from build123d import *

# Parameters (mm, degrees)
SKETCH1_R                    = 9
SKETCH1_R_2                  = 1
BOSS_EXTRUDE1_DEPTH          = 36
SKETCH5_W                    = 5
SKETCH5_H                    = 4.08502449
SKETCH5_W_2                  = 8
BOSS_EXTRUDE2_DEPTH          = 22
SKETCH7_W                    = 5
SKETCH7_H                    = 4.653899232
CUT_REVOLVE2_ANGLE           = 90
CUT_REVOLVE2_OTHER_WAY_ANGLE = 90
CIRPATTERN1_COUNT            = 15
SKETCH13_W                   = 5
SKETCH13_H                   = 16.616445935
SKETCH17_R                   = 2
CUT_EXTRUDE1_DEPTH           = 10
CUT_EXTRUDE2_DEPTH           = 23
CUT_EXTRUDE2_DEPTH_BACK      = 8
SKETCH20_R                   = 20.157813079
CUT_EXTRUDE3_DEPTH           = 36
FILLET1_R                    = 1


with BuildPart() as part:
    # Sketch1 → Boss-Extrude1 (new body)
    with BuildSketch(Plane.XY):
        Circle(SKETCH1_R)
        Circle(SKETCH1_R_2, mode=Mode.SUBTRACT)
    extrude(amount=BOSS_EXTRUDE1_DEPTH)

    # Sketch5 → Cut-Revolve1 (revolve, cut)
    with BuildSketch(Plane(origin=(0, 0, 0), x_dir=(0, 0, -1), z_dir=(1, 0, 0)), mode=Mode.PRIVATE) as cut_revolve1_sk:
        with Locations((-2.5, 6.957487755)):
            Rectangle(SKETCH5_W, SKETCH5_H)
        with Locations((-32, 6.957487755)):
            Rectangle(SKETCH5_W_2, SKETCH5_H)
    revolve(cut_revolve1_sk.sketch.rotate(Axis((0, 0, 0), (0, 0, 1)), 90), axis=Axis((0, 0, 0), (0, 0, 1)), mode=Mode.SUBTRACT)

    # Sketch6 → Boss-Extrude2 (add)
    with BuildSketch(Plane.XY):
        with BuildLine():
            Line((-1, 8.94427191), (-1, 10.94427191))
            ThreePointArc((-1, 10.94427191), (-0.927189817, 11.988569364), (-0.5, 12.94427191))
            Line((-0.5, 12.94427191), (0.5, 12.94427191))
            ThreePointArc((0.5, 12.94427191), (0.927189817, 11.988569364), (1, 10.94427191))
            Line((1, 10.94427191), (1, 8.94427191))
            Line((1, 8.94427191), (-1, 8.94427191))
        make_face()
    boss_extrude2 = extrude(amount=BOSS_EXTRUDE2_DEPTH)

    # Sketch7 → Cut-Revolve2 (revolve, cut)
    with BuildSketch(Plane(origin=(0, 0, 0), x_dir=(0, 0, -1), z_dir=(1, 0, 0))):
        with Locations((-2.5, 11.271221526)):
            Rectangle(SKETCH7_W, SKETCH7_H)
    revolve(axis=Axis((0, 8.94427191, 5), (0, 0, -1)), revolution_arc=CUT_REVOLVE2_ANGLE, mode=Mode.SUBTRACT)

    # Sketch7 → Cut-Revolve2 other way (revolve, cut)
    with BuildSketch(Plane(origin=(0, 0, 0), x_dir=(0, 0, -1), z_dir=(1, 0, 0))):
        with Locations((-2.5, 11.271221526)):
            Rectangle(SKETCH7_W, SKETCH7_H)
    revolve(axis=Axis((0, 8.94427191, 5), (0, 0, 1)), revolution_arc=CUT_REVOLVE2_OTHER_WAY_ANGLE, mode=Mode.SUBTRACT)

    # CirPattern1: Boss-Extrude2 ×15 about axis
    cirpattern1_axis = Axis((0, 0, 0), (0, 0, 1))
    for i in range(1, CIRPATTERN1_COUNT):
        add(boss_extrude2.rotate(cirpattern1_axis, i * 360 / CIRPATTERN1_COUNT))

    # Sketch13 → Cut-Revolve6 (revolve, cut)
    with BuildSketch(Plane(origin=(0, 0, 0), x_dir=(0, 0, -1), z_dir=(1, 0, 0)), mode=Mode.PRIVATE) as cut_revolve6_sk:
        with Locations((-2.5, 8.308222968)):
            Rectangle(SKETCH13_W, SKETCH13_H)
    revolve(cut_revolve6_sk.sketch.rotate(Axis((0, 0, 25.578402878), (0, 0, -1)), 270), axis=Axis((0, 0, 25.578402878), (0, 0, -1)), mode=Mode.SUBTRACT)

    # Sketch17 → Cut-Extrude1 (cut)
    with BuildSketch(Plane(origin=(0, 0, 0), x_dir=(1, 0, 0), z_dir=(0, 1, 0))):
        with Locations(Location((-0.128741976, -25.11123185, 0), (0, 0, 270))):
            Circle(SKETCH17_R)
    extrude(amount=-CUT_EXTRUDE1_DEPTH, mode=Mode.SUBTRACT)

    # Sketch20 → Cut-Extrude2 (cut, two sides: drawn at the far end of the back side and taken through both)
    with BuildSketch(Plane.XY.offset(28).offset(-CUT_EXTRUDE2_DEPTH_BACK)):
        Circle(SKETCH20_R)
    extrude(amount=CUT_EXTRUDE2_DEPTH + CUT_EXTRUDE2_DEPTH_BACK, mode=Mode.SUBTRACT)

    # Sketch21 → Cut-Extrude3 (cut)
    with BuildSketch(Plane.XY.offset(20)):
        Polygon((1.840953559, 2.223560956), (-1.005183496, 2.706093028), (-2.846137055, 0.482532071), (-1.840953559, -2.223560956), (1.005183496, -2.706093028), (2.846137055, -0.482532071), align=None)
    extrude(amount=-CUT_EXTRUDE3_DEPTH, mode=Mode.SUBTRACT)

    # Fillet1
    fillet1_edges = [part.edges().sort_by_distance(p)[0] for p in [
        (2.343545307, 0.870514443, 5),
        (1.925660275, -1.594312549, 5),
        (-0.417885032, -2.464826992, 5),
        (-2.343545307, -0.870514443, 5),
        (-1.925660275, 1.594312549, 5),
        (0.417885032, 2.464826992, 5),
        (2.343545307, 0.870514443, 20),
        (0.417885032, 2.464826992, 20),
        (-1.925660275, 1.594312549, 20),
        (-2.343545307, -0.870514443, 20),
        (-0.417885032, -2.464826992, 20),
        (1.925660275, -1.594312549, 20),
    ]]
    fillet(fillet1_edges, radius=FILLET1_R)


solid = part.part
The listing builds one solid part. Answer for the finished solid, in the listing's coordinates (mm). A direction names the side the tool comes from. Coordinates: 2 decimals unless noted, no trailing zeros.
1) Find the intervals of material crossed by L1, parallel to X at y = 10.5, z = 19.5; L2, parallel to X at y = -10, z = 10.25; L3, parallel to Y at x = 7.5, z = 14.25, in increasing order.
2) Determine the mould class of faces 1 (the face through (11.21, -6.47, 12.4)), 2 (the face through (-5.271, 11.822, 12.395)), 3 (the face through (-11.13, 4.587, 12.395)) for opening direction X: pulls with the +X half, pulls with the -X half, needs draft (parallel to the pull), parting line crosses it, or undercut.
3) Flat-ended cylindrical pins translate along their axes: pin 1 Ø4 at (x, z) = (0, 18) entering from -Y; pin 2 Ø4 at (x, z) = (9, 11.5) entering from -Y; pin 3 Ø0.6 at (y, z) = (10.5, 12) entering from -X. Find the tip coordinate at first contact, or state that the pin passes through.
4) A tool of negligible diameter and unlimited length cuts with its end or side. For faces 4 (the face through (-9.771, -2.033, 12.395)), 5 (the face through (0.44, 2.766, 5.285)), 6 (the face through (-2.6, -1, 19.7)), 7 (the face through (7.79, -9.14, 12.4)), from which of +Z, -Z, +X, -X, +Y, -Y can it reach the whole face along a straight path? Write none if from no direction.
Values:
1. L1: x = -5.71 to -3.57, -1 to 1, 3.57 to 5.71
1. L2: x = -8 to -6.04, -3.15 to -1.1, 1.1 to 3.15, 6.04 to 8
1. L3: y = -10.55 to -8.6, -5.48 to 4.97, 5.41 to 8.11
2. face 1: pulls with the +X half
2. face 2: pulls with the -X half
2. face 3: undercut
3. pin 1: stops at y = -12.55
3. pin 2: stops at y = -10.77
3. pin 3: stops at x = -5.75
4. face 4: +Z, -Z
4. face 5: -Z
4. face 6: +Z
4. face 7: +Z, -Z, +X
